Check sheet for the modelled part. Datum: model origin and axes. Units: mm. Face numbers are marked on the shaded views. Round coordinates to 2 decimals unless told otherwise and drop trailing zeros. Order: outer loops, then holes, each group sorted by start corner. A loop starts at its lowest first (then second) coordinate and runs counter-clockwise, first axis right, second up.
(1) Sectioned sample at B-B, the plane y = -25. Enter the section's corners in (x, z) (1 decimal).
(2) Mould release check, pull along X, two halves, no side actions. Record for the marked faces 1 and 2: released by +X, released by -X, zero draft, split by the parting line, or undercut.
(3) Depth check by flat-ended pin: pin 1 (1.6 mm diameter, centred on y = -25.5, z = -1, fed in from -X); pin 2 (0.7 mm diameter, centred on y = 48, z = -1, fed in from -X); pin 3 (1.8 mm diameter, centred on y = -13.5, z = -5, fed in from +X). Enter the tip coordinate at first touch or a pass-through.
(4) Sectioned sample at A-A, the plane x = 0. Enter the section's corners in (y, z) (3 decimals), and give its area (3 significant figures).
(5) Thickness scan on probe 1 along X at (y, z) = (-10, -2.5); probe 2 along Z at (x, y) = (3, 39.5); probe 3 along X at (y, z) = (-15, -2). Record the ranges inside material, lowest first.
(6) Sectioned sample at C-C, the plane z = -5. Enter the section's corners in (x, y) (1 decimal).
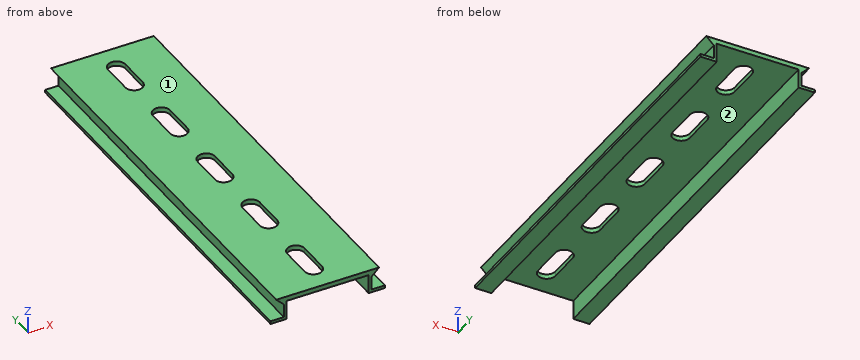
```python
from build123d import *

# Parameters (mm, degrees)
BOSS_EXTRUDE1_DEPTH = 62.865
CUT_EXTRUDE1_DEPTH  = 66.710688552


with BuildPart() as part:
    # Sketch1 → Boss-Extrude1 (new, symmetric)
    with BuildSketch(Plane(origin=(0, 0, 0), x_dir=(1, 0, 0), z_dir=(0, 1, 0))):
        Polygon((-15.875, 0), (0, 0), (0, 1.4478), (-12.6365, 1.4478), (-12.6365, 7.366), (-17.653, 7.366), (-17.653, 6.477), (-13.5255, 6.477), (-13.5255, 2.286), align=None)
        Polygon((0, 1.4478), (0, 0), (15.875, 0), (13.5255, 2.286), (13.5255, 6.477), (17.653, 6.477), (17.653, 7.366), (12.6365, 7.366), (12.6365, 1.4478), align=None)
    extrude(amount=BOSS_EXTRUDE1_DEPTH, both=True)

    # Sketch2 → Cut-Extrude1 (cut, through all)
    with BuildSketch(Plane.XY):
        with BuildLine():
            Line((-2.667, -4.833), (-2.667, 4.833))
            ThreePointArc((-2.667, 4.833), (0, 7.5), (2.667, 4.833))
            Line((2.667, 4.833), (2.667, -4.833))
            ThreePointArc((2.667, -4.833), (0, -7.5), (-2.667, -4.833))
        make_face()
        with BuildLine():
            Line((-2.667, 20.167), (-2.667, 29.833))
            ThreePointArc((-2.667, 29.833), (0, 32.5), (2.667, 29.833))
            Line((2.667, 29.833), (2.667, 20.167))
            ThreePointArc((2.667, 20.167), (0, 17.5), (-2.667, 20.167))
        make_face()
        with BuildLine():
            Line((-2.667, 45.167), (-2.667, 54.833))
            ThreePointArc((-2.667, 54.833), (0, 57.5), (2.667, 54.833))
            Line((2.667, 54.833), (2.667, 45.167))
            ThreePointArc((2.667, 45.167), (0, 42.5), (-2.667, 45.167))
        make_face()
        with BuildLine():
            Line((-2.667, -29.833), (-2.667, -20.167))
            ThreePointArc((-2.667, -20.167), (0, -17.5), (2.667, -20.167))
            Line((2.667, -20.167), (2.667, -29.833))
            ThreePointArc((2.667, -29.833), (0, -32.5), (-2.667, -29.833))
        make_face()
        with BuildLine():
            Line((-2.667, -54.833), (-2.667, -45.167))
            ThreePointArc((-2.667, -45.167), (0, -42.5), (2.667, -45.167))
            Line((2.667, -45.167), (2.667, -54.833))
            ThreePointArc((2.667, -54.833), (0, -57.5), (-2.667, -54.833))
        make_face()
    extrude(amount=-CUT_EXTRUDE1_DEPTH, mode=Mode.SUBTRACT)


solid = part.part
```
Derived:
1. outline: (-17.7, -7.4) - (-12.6, -7.4) - (-12.6, -1.4) - (-2.7, -1.4) - (-2.7, 0) - (-15.9, 0) - (-13.5, -2.3) - (-13.5, -6.5) - (-17.7, -6.5) - close; (2.7, -1.4) - (12.6, -1.4) - (12.6, -7.4) - (17.7, -7.4) - (17.7, -6.5) - (13.5, -6.5) - (13.5, -2.3) - (15.9, 0) - (2.7, 0) - close
2. face 1: zero draft
2. face 2: undercut
3. pin 1: stops at x = -15.67
3. pin 2: stops at x = -15.21
3. pin 3: stops at x = 13.53
4. outline: (-62.865, -1.448) - (-57.5, -1.448) - (-57.5, 0) - (-62.865, 0) - close; (-42.5, -1.448) - (-32.5, -1.448) - (-32.5, 0) - (-42.5, 0) - close; (-17.5, -1.448) - (-7.5, -1.448) - (-7.5, 0) - (-17.5, 0) - close; (7.5, -1.448) - (17.5, -1.448) - (17.5, 0) - (7.5, 0) - close; (32.5, -1.448) - (42.5, -1.448) - (42.5, 0) - (32.5, 0) - close; (57.5, -1.448) - (62.865, -1.448) - (62.865, 0) - (57.5, 0) - close
4. area: 73.4 mm2
5. probe 1: x = -13.53 to -12.64, 12.64 to 13.53
5. probe 2: z = -1.45 to 0
5. probe 3: x = -13.82 to -12.64, 12.64 to 13.82
6. outline: (-13.5, -62.9) - (-12.6, -62.9) - (-12.6, 62.9) - (-13.5, 62.9) - close; (12.6, -62.9) - (13.5, -62.9) - (13.5, 62.9) - (12.6, 62.9) - close
